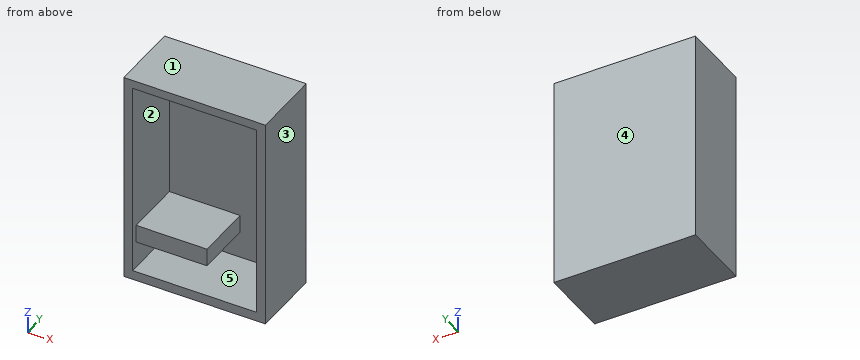
from build123d import *

# Parameters (mm, degrees)
F0_W     = 50.8
F0_H     = 76.2
F1_DEPTH = 25.4
F2_W     = 44.45
F2_H     = 69.85
F3_DEPTH = 22.86
F4_W     = 22.86
F4_H     = 6.35
F5_DEPTH = 25.4


with BuildPart() as f1:
    # F0 (on Front) → F1 (new body)
    with BuildSketch(Plane.XZ):
        with Locations((-25.4, 38.1)):
            Rectangle(F0_W, F0_H)
    extrude(amount=F1_DEPTH)

    # F2 (on face) → F3 (cut)
    with BuildSketch(Plane.XZ.offset(25.4)):
        with Locations((-25.384539, 38.258707)):
            Rectangle(F2_W, F2_H)
    extrude(amount=-F3_DEPTH, mode=Mode.SUBTRACT)

    # F4 (on face) → F5 (join)
    with BuildSketch(Plane.YZ.offset(-47.609539)):
        with Locations((-11.782601, 16.132223)):
            Rectangle(F4_W, F4_H)
    extrude(amount=F5_DEPTH)


solid = f1.part
Build history of the part. All positions in model axes, mm. Face numbers are marked on the shaded views. A direction names the side the tool comes from. Round coordinates to 2 decimals unless told otherwise and drop trailing zeros. Loops run counter-clockwise (first coordinate to the right, second up) from the corner with the lowest first, then second, coordinate; pieces in that order, holes last. Notation, with made-up numbers: (31.5, 21.25) -> (43.5, 21.25) arc R12 cw to (43.5, 34.25) -> close; hole circle Ø7 at (65.5, 77). An arc over 180 degrees is marked (long way). One line per item, written item: value. Start each with the question number.
Q1. Two-plate mould, pull along X, no slides. Class the marked faces 1, 2 and 3: released by +X, released by -X, zero draft, split by the parting line, or undercut.
Q2. Probe line 1 along Z through (x, y) = (-29, -8.75); line 2 along Z through (x, y) = (-19, -13.25); line 3 along X through (y, z) = (-6.5, 34.5). List the from-to ranges inside material, lowest first.
Q3. Cut at C-C on z = 41. List the corners of the cut face in (x, y), plus the area to 3 significant figures.
Q4. 3-axis set-ups, long thin cutter, end or side, ignore diameter. For the marked faces 4 and 5: which of +Z, -Z, +X, -X, +Y, -Y reach the whole face in a straight line?
Q5. Cut at B-B on x = -11. List the corners of the cut face in (y, z), plus the area to 3 significant figures.
Q6. Cut at A-A on y = -5.5. List the corners of the cut face in (x, z), plus the area to 3 significant figures.
Q7. Cut at D-D on x = -24.5. List the corners of the cut face in (y, z), plus the area to 3 significant figures.
Q8. Drop flat-ended pins along their axis: pin 1 Ø12 at (x, y) = (-18.5, -20.5) entering from -Z; pin 2 Ø1 at (x, z) = (-5.5, 33) entering from -Y; pin 3 Ø5 at (x, z) = (-33.5, 16) entering from -Y. Give the stop position or say it passes through.
Computed:
1. face 1: zero draft
1. face 2: undercut
1. face 3: released by +X
2. line 1: 0 to 3.33, 12.96 to 19.31, 73.18 to 76.2
2. line 2: 0 to 3.33, 73.18 to 76.2
2. line 3: -50.8 to -47.61, -3.16 to 0
3. outline: (-50.8, -25.4) -> (-47.61, -25.4) -> (-47.61, -2.54) -> (-3.16, -2.54) -> (-3.16, -25.4) -> (0, -25.4) -> (0, 0) -> (-50.8, 0) -> close
3. area: 274 mm²
4. face 4: +Z, -Z, +X, -X, +Y
4. face 5: -Y
5. outline: (-25.4, 0) -> (0, 0) -> (0, 76.2) -> (-25.4, 76.2) -> (-25.4, 73.18) -> (-2.54, 73.18) -> (-2.54, 3.33) -> (-25.4, 3.33) -> close
5. area: 339 mm²
6. outline: (-50.8, 0) -> (0, 0) -> (0, 76.2) -> (-50.8, 76.2) -> close; hole (-47.61, 3.33) -> (-3.16, 3.33) -> (-3.16, 73.18) -> (-47.61, 73.18) -> (-47.61, 19.31) -> (-22.21, 19.31) -> (-22.21, 12.96) -> (-47.61, 12.96) -> close
6. area: 927 mm²
7. outline: (-25.4, 0) -> (0, 0) -> (0, 76.2) -> (-25.4, 76.2) -> (-25.4, 73.18) -> (-2.54, 73.18) -> (-2.54, 19.31) -> (-23.21, 19.31) -> (-23.21, 12.96) -> (-2.54, 12.96) -> (-2.54, 3.33) -> (-25.4, 3.33) -> close
7. area: 470 mm²
8. pin 1: z = 0
8. pin 2: y = -2.54
8. pin 3: y = -23.21
